Source: CAD feature listing. Evaluate the final solid. Frame: model axes, mm. A direction names the side the tool comes from. Round coordinates to 2 decimals unless told otherwise and drop trailing zeros. Write each loop counter-clockwise with the first axis right and the second up, starting at its lowest first coordinate (ties: lowest second). Pieces come first, ordered by that corner, then holes.
from build123d import *

# Parameters (mm, degrees)
SKETCH1_W                = 170
SKETCH1_H                = 130
BOSS_EXTRUDE1_DEPTH      = 8
SKETCH2_R                = 1.5
SKETCH2_W                = 165
SKETCH2_H                = 100
CUT_EXTRUDE1_DEPTH       = 21
SKETCH3_W                = 170
SKETCH3_H                = 20
BOSS_EXTRUDE2_DEPTH      = 8
SKETCH4_W                = 65
SKETCH4_H                = 16.2
CUT_EXTRUDE2_DEPTH       = 2
SKETCH5_W                = 3.5
SKETCH5_H                = 12
CUT_EXTRUDE3_DEPTH       = 35
SKETCH6_W                = 170
SKETCH6_H                = 150
BOSS_EXTRUDE3_DEPTH      = 8
BOSS_EXTRUDE4_DEPTH      = 138
SKETCH8_W                = 249
SKETCH8_H                = 138
BOSS_EXTRUDE5_DEPTH      = 1
SKETCH9_W                = 72.8
SKETCH9_H                = 73.25
CUT_EXTRUDE4_DEPTH       = 19
BOSS_EXTRUDE6_DEPTH      = 5
SKETCH11_R               = 1.5
CUT_EXTRUDE5_DEPTH       = 56
SKETCH12_R               = 9
SKETCH12_R_2             = 6.5
SKETCH12_R_3             = 1
SKETCH12_R_4             = 2.75
CUT_EXTRUDE6_DEPTH       = 115
SKETCH13_W               = 58.59049163
SKETCH13_H               = 30.075830986
CUT_EXTRUDE7_DEPTH       = 3
FILLET1_R                = 2
SKETCH15_R               = 1.5
CUT_EXTRUDE8_DEPTH       = 10
CUT_EXTRUDE10_DEPTH      = 261
SKETCH19_R               = 1.5
BOSS_EXTRUDE7_DEPTH      = 8
BOSS_EXTRUDE12_START     = -124.5
BOSS_EXTRUDE12_DEPTH     = 249
SKETCH22_R               = 1.5
SKETCH22_W               = 165
SKETCH22_H               = 100
CUT_EXTRUDE11_DEPTH      = 18
FILLET2_R                = 10
SKETCH24_R               = 2
SKETCH24_W               = 3
SKETCH24_H               = 72
CUT_EXTRUDE15_DEPTH      = 42
CUT_EXTRUDE16_DEPTH      = 140
CUT_EXTRUDE16_DEPTH_BACK = 242
SKETCH27_W               = 249
SKETCH27_H               = 105
BOSS_EXTRUDE13_DEPTH     = 7
CUT_EXTRUDE17_DEPTH      = 249
FILLET6_R                = 3
FILLET7_R                = 3
BOSS_EXTRUDE14_DEPTH     = 9
SKETCH30_R               = 1.5
CUT_EXTRUDE18_DEPTH      = 10
SKETCH31_R               = 1.5
CUT_EXTRUDE19_DEPTH      = 49
CUT_EXTRUDE20_DEPTH      = 49


with BuildPart() as part:
    # Sketch1 → Boss-Extrude1 (new body)
    with BuildSketch(Plane.XY):
        with Locations((85, 65)):
            Rectangle(SKETCH1_W, SKETCH1_H)
    extrude(amount=BOSS_EXTRUDE1_DEPTH)

    # Sketch2 → Cut-Extrude1 (cut)
    with BuildSketch(Plane.XY.offset(8)):
        with Locations((6.55, 123.35)):
            Circle(SKETCH2_R)
        with Locations((163.45, 123.35)):
            Circle(SKETCH2_R)
        with Locations((6.55, 6.65)):
            Circle(SKETCH2_R)
        with Locations((163.45, 6.65)):
            Circle(SKETCH2_R)
        with Locations((85, 65)):
            Rectangle(SKETCH2_W, SKETCH2_H)
    extrude(amount=-CUT_EXTRUDE1_DEPTH, mode=Mode.SUBTRACT)

    # Sketch3 → Boss-Extrude2 (add)
    with BuildSketch(Plane.XY.offset(8)):
        with Locations((85, -10)):
            Rectangle(SKETCH3_W, SKETCH3_H)
    extrude(amount=-BOSS_EXTRUDE2_DEPTH)

    # Sketch4 → Cut-Extrude2 (cut)
    with BuildSketch(Plane.XY.offset(8)):
        with Locations((85, -10)):
            Rectangle(SKETCH4_W, SKETCH4_H)
    extrude(amount=-CUT_EXTRUDE2_DEPTH, mode=Mode.SUBTRACT)

    # Sketch5 → Cut-Extrude3 (cut)
    with BuildSketch(Plane.XY.offset(6)):
        with Locations((63.25, -10)):
            Rectangle(SKETCH5_W, SKETCH5_H)
        with Locations((71.75, -10)):
            Rectangle(SKETCH5_W, SKETCH5_H)
        with Locations((80.75, -10)):
            Rectangle(SKETCH5_W, SKETCH5_H)
        with Locations((89.25, -10)):
            Rectangle(SKETCH5_W, SKETCH5_H)
        with Locations((98.25, -10)):
            Rectangle(SKETCH5_W, SKETCH5_H)
        with Locations((106.75, -10)):
            Rectangle(SKETCH5_W, SKETCH5_H)
    extrude(amount=-CUT_EXTRUDE3_DEPTH, mode=Mode.SUBTRACT)

    # Sketch6 → Boss-Extrude3 (add)
    with BuildSketch(Plane.XY.offset(8)):
        Polygon((15.504384948, 140), (225, 140), (225, -35), (-10, -35), (-10, 140), align=None)
        with Locations((85, 55)):
            Rectangle(SKETCH6_W, SKETCH6_H, mode=Mode.SUBTRACT)
    extrude(amount=-BOSS_EXTRUDE3_DEPTH)

    # Sketch7 → Boss-Extrude4 (add)
    with BuildSketch(Plane.XY.offset(8)):
        Polygon((-10, 140), (-17, 140), (-17, -42), (232, -42), (232, 140), (225, 140), (225, -35), (-10, -35), align=None)
    extrude(amount=-BOSS_EXTRUDE4_DEPTH)

    # Sketch8 → Boss-Extrude5 (add)
    with BuildSketch(Plane.XZ.offset(42)):
        with Locations((107.5, -61)):
            Rectangle(SKETCH8_W, SKETCH8_H)
    extrude(amount=BOSS_EXTRUDE5_DEPTH)

    # Sketch9 → Cut-Extrude4 (cut)
    with BuildSketch(Plane(origin=(232, 0, 0), x_dir=(0, 0, -1), z_dir=(1, 0, 0))):
        with Locations((75, 35)):
            Rectangle(SKETCH9_W, SKETCH9_H)
    extrude(amount=-CUT_EXTRUDE4_DEPTH, mode=Mode.SUBTRACT)

    # Sketch10 → Boss-Extrude6 (add)
    with BuildSketch(Plane(origin=(232, 0, 0), x_dir=(0, 0, -1), z_dir=(1, 0, 0))):
        Polygon((36, 44), (36, -4), (114, -4), (114, 44), (119, 44), (119, -9), (31, -9), (31, 44), align=None)
    extrude(amount=BOSS_EXTRUDE6_DEPTH)

    # Sketch11 → Cut-Extrude5 (cut)
    with BuildSketch(Plane(origin=(237, 0, 0), x_dir=(0, 0, -1), z_dir=(1, 0, 0))):
        with Locations((33.5, 17.5)):
            Circle(SKETCH11_R)
        with Locations((116.5, 17.5)):
            Circle(SKETCH11_R)
    extrude(amount=-CUT_EXTRUDE5_DEPTH, mode=Mode.SUBTRACT)

    # Sketch12 → Cut-Extrude6 (cut)
    with BuildSketch(Plane(origin=(0, -35, 0), x_dir=(1, 0, 0), z_dir=(0, 1, 0))):
        with Locations(Location((166.25, 32.5, 0), (0, 0, 180))):
            Circle(SKETCH12_R)
        with Locations(Location((166.25, 97.5, 0), (0, 0, 180))):
            Circle(SKETCH12_R_2)
        with Locations(Location((155.75, 97.5, 0), (0, 0, 180))):
            Circle(SKETCH12_R_3)
        with Locations(Location((155.75, 85, 0), (0, 0, 180))):
            Circle(SKETCH12_R_3)
        with Locations(Location((176.75, 85, 0), (0, 0, 180))):
            Circle(SKETCH12_R_3)
        with Locations(Location((176.75, 97.5, 0), (0, 0, 180))):
            Circle(SKETCH12_R_3)
        with Locations(Location((145.25, 97.5, 0), (0, 0, 180))):
            Circle(SKETCH12_R_4)
        with Locations(Location((187.25, 97.5, 0), (0, 0, 180))):
            Circle(SKETCH12_R_4)
    extrude(amount=-CUT_EXTRUDE6_DEPTH, mode=Mode.SUBTRACT)

    # Sketch13 → Cut-Extrude7 (cut)
    with BuildSketch(Plane.XZ.offset(43)):
        with Locations((166.25, -93.48757215)):
            Rectangle(SKETCH13_W, SKETCH13_H)
    extrude(amount=-CUT_EXTRUDE7_DEPTH, mode=Mode.SUBTRACT)

    # Fillet1
    fillet1_edges = [part.edges().sort_by_distance(p)[0] for p in [
        (136.954754185, -40, -93.48757215),
        (166.25, -40, -78.449656657),
        (195.545245815, -40, -93.48757215),
        (166.25, -40, -108.525487643),
    ]]
    fillet(fillet1_edges, radius=FILLET1_R)

    # Sketch15 → Cut-Extrude8 (cut)
    with BuildSketch(Plane(origin=(0, 140, 0), x_dir=(1, 0, 0), z_dir=(0, 1, 0))):
        with Locations(Location((5, -4, 0), (0, 0, 270))):
            Circle(SKETCH15_R)
        with Locations(Location((20, -4, 0), (0, 0, 270))):
            Circle(SKETCH15_R)
        with Locations(Location((217, -4, 0), (0, 0, 90))):
            Circle(SKETCH15_R)
        with Locations(Location((202, -4, 0), (0, 0, 90))):
            Circle(SKETCH15_R)
    extrude(amount=-CUT_EXTRUDE8_DEPTH, mode=Mode.SUBTRACT)

    # Sketch18 → Cut-Extrude10 (cut)
    with BuildSketch(Plane(origin=(232, 0, 0), x_dir=(0, 0, -1), z_dir=(1, 0, 0))):
        Polygon((45.496279283, 140), (-8, 140), (-8, 15), (0, 15), align=None)
    extrude(amount=-CUT_EXTRUDE10_DEPTH, mode=Mode.SUBTRACT)

    # Sketch19 → Boss-Extrude7 (add)
    with BuildSketch(Plane.XY.offset(8)):
        with Locations((6.55, 6.65)):
            Circle(SKETCH19_R)
        with Locations((163.45, 6.65)):
            Circle(SKETCH19_R)
    extrude(amount=-BOSS_EXTRUDE7_DEPTH)

    # Sketch21 → Boss-Extrude12 (add)
    with BuildSketch(Plane(origin=(107.5, 0, 0), x_dir=(0, 0, -1), z_dir=(1, 0, 0)).offset(BOSS_EXTRUDE12_START)):
        Polygon((45.496279283, 140), (0, 15), (-8, 15), (37.496279283, 140), align=None)
    extrude(amount=BOSS_EXTRUDE12_DEPTH)

    # Sketch22 → Cut-Extrude11 (cut)
    with BuildSketch(Plane(origin=(0, 4.325817115, 11.885084845), x_dir=(1, 0, 0), z_dir=(0, 0.3420201433256603, 0.9396926207859115))):
        with Locations(Location((1.55, 136.220338945, 0), (0, 0, 270))):
            Circle(SKETCH22_R)
        with Locations(Location((158.45, 136.220338945, 0), (0, 0, 270))):
            Circle(SKETCH22_R)
        with Locations(Location((1.55, 19.520338945, 0), (0, 0, 270))):
            Circle(SKETCH22_R)
        with Locations(Location((158.45, 19.520338945, 0), (0, 0, 270))):
            Circle(SKETCH22_R)
        with Locations((80, 77.870338945)):
            Rectangle(SKETCH22_W, SKETCH22_H)
    extrude(amount=-CUT_EXTRUDE11_DEPTH, mode=Mode.SUBTRACT)

    # Fillet2
    fillet2_edges = [part.edges().sort_by_distance(p)[0] for p in [
        (107.5, 15, 8),
    ]]
    fillet(fillet2_edges, radius=FILLET2_R)

    # Sketch24 → Cut-Extrude15 (cut)
    with BuildSketch(Plane(origin=(-10, 0, 0), x_dir=(0, 0, -1), z_dir=(1, 0, 0))):
        with Locations(Location((113.5, 48.5, 0), (0, 0, 90))):
            Circle(SKETCH24_R)
        with Locations(Location((119.5, 68.5, 0), (0, 0, 90))):
            Circle(SKETCH24_R)
        with Locations(Location((119.5, 28.5, 0), (0, 0, 90))):
            Circle(SKETCH24_R)
        with Locations((128.5, 48.5)):
            Rectangle(SKETCH24_W, SKETCH24_H)
    extrude(amount=-CUT_EXTRUDE15_DEPTH, mode=Mode.SUBTRACT)

    # Sketch25 → Cut-Extrude16 (cut, two sides: drawn at the far end of the back side and taken through both)
    with BuildSketch(Plane(origin=(232, 0, 0), x_dir=(0, 0, -1), z_dir=(1, 0, 0)).offset(-CUT_EXTRUDE16_DEPTH_BACK)):
        Polygon((45.496279283, 140), (130, 140), (130, -43), (0, -43), (0, 15), align=None)
    extrude(amount=CUT_EXTRUDE16_DEPTH + CUT_EXTRUDE16_DEPTH_BACK, mode=Mode.SUBTRACT)

    # Sketch27 → Boss-Extrude13 (add)
    with BuildSketch(Plane(origin=(0, 140, 0), x_dir=(1, 0, 0), z_dir=(0, 1, 0))):
        with Locations((107.5, 89.996279283)):
            Rectangle(SKETCH27_W, SKETCH27_H)
    extrude(amount=BOSS_EXTRUDE13_DEPTH)

    # Sketch28 → Cut-Extrude17 (cut)
    with BuildSketch(Plane(origin=(232, 0, 0), x_dir=(0, 0, -1), z_dir=(1, 0, 0))):
        Polygon((37.496279283, 140), (40.044070923, 147), (37.496279283, 147), align=None)
    extrude(amount=-CUT_EXTRUDE17_DEPTH, mode=Mode.SUBTRACT)

    # Fillet6
    fillet6_edges = [part.edges().sort_by_distance(p)[0] for p in [
        (107.5, 140, -142.496279283),
    ]]
    fillet(fillet6_edges, radius=FILLET6_R)

    # Fillet7
    fillet7_edges = [part.edges().sort_by_distance(p)[0] for p in [
        (-17, 145, -142.496279283),
        (-17, 140, -134.748139642),
        (-17, 140.878679656, -141.617599627),
    ]]
    fillet(fillet7_edges, radius=FILLET7_R)

    # Sketch29 → Boss-Extrude14 (add)
    with BuildSketch(Plane(origin=(232, 0, 0), x_dir=(0, 0, -1), z_dir=(1, 0, 0))):
        with BuildLine():
            Line((-8, -43), (0, -43))
            Line((0, -43), (0, 15))
            Line((0, 15), (45.496279283, 140))
            Line((45.496279283, 140), (139.496279283, 140))
            ThreePointArc((139.496279283, 140), (141.886652657, 140.990125071), (142.876777727, 143.380498444))
            Line((142.876777727, 143.380498444), (142.496279283, 147))
            Line((142.496279283, 147), (40.044070923, 147))
            Line((40.044070923, 147), (-7.396926208, 16.656931626))
            ThreePointArc((-7.396926208, 16.656931626), (-7.84807753, 14.97321197), (-8, 13.236730193))
            Line((-8, 13.236730193), (-8, -43))
        make_face()
    extrude(amount=BOSS_EXTRUDE14_DEPTH)

    # Sketch30 → Cut-Extrude18 (cut)
    with BuildSketch(Plane(origin=(0, 147, 0), x_dir=(1, 0, 0), z_dir=(0, 1, 0))):
        with Locations(Location((218.25, 136.876777727, 0), (0, 0, 270))):
            Circle(SKETCH30_R)
        with Locations(Location((203.25, 136.876777727, 0), (0, 0, 270))):
            Circle(SKETCH30_R)
    extrude(amount=-CUT_EXTRUDE18_DEPTH, mode=Mode.SUBTRACT)

    # Sketch31 → Cut-Extrude19 (cut)
    with BuildSketch(Plane.XY.offset(8)):
        with Locations((219, -39)):
            Circle(SKETCH31_R)
        with Locations((204, -39)):
            Circle(SKETCH31_R)
    extrude(amount=-CUT_EXTRUDE19_DEPTH, mode=Mode.SUBTRACT)

    # Sketch32 → Cut-Extrude20 (cut)
    with BuildSketch(Plane.ZY.offset(17)):
        with BuildLine():
            Line((-110, 0.736730193), (-12, 0.736730193))
            ThreePointArc((-12, 0.736730193), (-4.5, -6.763269807), (-12, -14.263269807))
            Line((-12, -14.263269807), (-110, -14.263269807))
            ThreePointArc((-110, -14.263269807), (-117.5, -6.763269807), (-110, 0.736730193))
        make_face()
        with BuildLine():
            Line((-110, 119.5), (-48.588668173, 119.5))
            ThreePointArc((-48.588668173, 119.5), (-41.088668173, 112), (-48.588668173, 104.5))
            Line((-48.588668173, 104.5), (-110, 104.5))
            ThreePointArc((-110, 104.5), (-117.5, 112), (-110, 119.5))
        make_face()
    extrude(amount=-CUT_EXTRUDE20_DEPTH, mode=Mode.SUBTRACT)


solid = part.part
1) Section query A-A on z = -56. Return the cut outline in (x, y).
Taken from the geometry:
outline: (-17, -43) - (-10, -43) - (-10, -14.26) - (-17, -14.26) - close; (-17, 0.74) - (-10, 0.74) - (-10, 104.5) - (-17, 104.5) - close; (-17, 119.5) - (-10, 119.5) - (-10, 140) - (241, 140) - (241, 147) - (-17, 147) - close
2) Contact query for flat-ended pins moving along their axis: P1, Ø2, axis at x = -15, y = 50.5, coming from the -Z side; P2, Ø2, axis at x = 210.5, z = -77.5, coming from the -Y side; P3, Ø10, axis at x = 164.5, y = 104, coming from the +Z side. Output: stop coordinate, or through.
Taken from the geometry:
P1: stops at z = -127
P2: stops at y = 140
P3: stops at z = -22.57
3) Reachability of faces 4 (the face through (-14, 104.5, -79)), 5 (the face through (61.5, -10, 3)), 6 (the face through (-10, 47, -64)), 7 (the face through (-14, -15, -130)) from +Z, -Z, +X, -X, +Y, -Y: full face, straight path, thin tool, end or side. Return the list, or none.
Taken from the geometry:
face 4: +X, -X
face 5: +Z, -Z
face 6: -Z, +X, -Y
face 7: -Z, +X, -X, -Y
4) Pull-direction query (Z, two-part tool) for faces 1 (the face through (105, -10, 3)), 2 (the face through (-13.5, -6.6, -4.5)), 3 (the face through (78.845, 123.217, -35.332)); classes: released by +Z, released by -Z, zero draft, split by the parting line, or undercut.
Taken from the geometry:
face 1: zero draft
face 2: undercut
face 3: released by +Z
5) Section query C-C on y = 112. Return the cut outline in (x, z), then the cut area to 3 significant figures.
Taken from the geometry:
outline: (-17, -130) - (-10, -130) - (-10, -117.5) - (-17, -117.5) - close; (-17, -41.09) - (-10, -41.09) - (-10, -35.31) - (-2.5, -35.31) - (-2.5, -27.31) - (-17, -27.31) - close; (162.5, -35.31) - (241, -35.31) - (241, -27.31) - (162.5, -27.31) - close
area: 872 mm2
6) Section query B-B on x = 20.5. Return the cut outline in (y, z), then the cut area to 3 significant figures.
Taken from the geometry:
outline: (-43, 0) - (15, 0) - (27.94, -4.71) - (30.52, 2.35) - (16.66, 7.4) arc R10 ccw to (13.24, 8) - (-43, 8) - close; (121.91, -38.91) - (140, -45.5) - (140, -139.5) arc R3 ccw to (143, -142.5) - (147, -142.5) - (147, -40.04) - (124.48, -31.85) - close
area: 1,440 mm2
7) Material intervals for line 1 (Z direction, x = 114.5, y = 1); line 2 (Y direction, x = 1, z = -78.5); line 3 (X direction, y = 65, z = -98), sorted ascending.
Taken from the geometry:
line 1: z = 0 to 8
line 2: y = 140 to 147
line 3: x = -17 to -10
